Read the model definition and answer for the solid it produces. Units are mm, in the model's axes. Face numbers are marked on the shaded views. Coordinates: 2 decimals unless noted, no trailing zeros. Write each loop counter-clockwise with the first axis right and the second up, starting at its lowest first coordinate (ties: lowest second). Pieces come first, ordered by that corner, then holes. Notation, with made-up numbers: (-5, 20.5) -> (13, 20.5) arc R19 cw to (13, 51.5) -> close; hole circle Ø9 at (44, 12). An arc over 180 degrees is marked (long way). One line per item, written item: value. Start each with the question number.
from build123d import *

# Parameters (mm, degrees)
F0_R     = 9.8
F0_R_2   = 9.65
F1_DEPTH = 4
F2_DEPTH = 3
F3_R     = 0.2


with BuildPart() as f1:
    # F0 (on Top) → F1 (new body)
    with BuildSketch(Plane.XY):
        Circle(F0_R)
        Circle(F0_R_2, mode=Mode.SUBTRACT)
        Circle(F0_R_2)
    extrude(amount=F1_DEPTH)

    # F0 (on Top) → F2 (cut)
    with BuildSketch(Plane.XY):
        Circle(F0_R_2)
    extrude(amount=F2_DEPTH, mode=Mode.SUBTRACT)

    # F3
    f3_edges = [f1.edges().sort_by_distance(p)[0] for p in [
        (-9.8, 0, 4),
        (-9.65, 0, 3),
    ]]
    fillet(f3_edges, radius=F3_R)


solid = f1.part
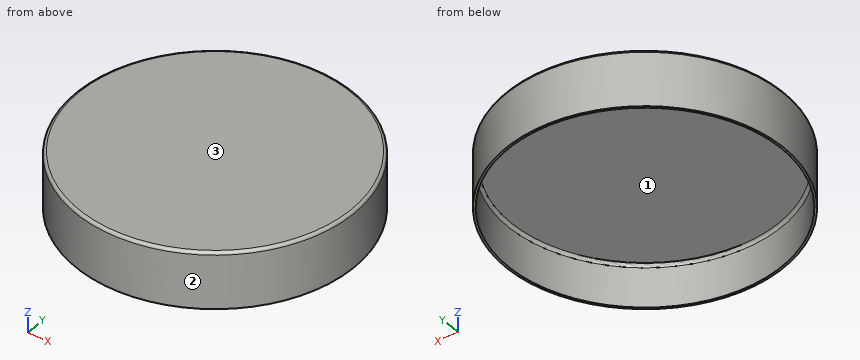
1. A cutting plane is placed at A-A on x = 0. Give the vertices of the cut face in (y, z).
2. For a pull along X with two mould halves and no side action, classify the marked faces 1, 2 and 3 as +X half, -X half, draft (parallel to the pull), parting line (faces both ways), or undercut.
3. Find the intervals of material crossed by probe 1 along Z at (x, y) = (6.5, 3.5); probe 2 along X at (y, z) = (-0.25, 2.65); probe 3 along X at (y, z) = (-8.5, 2.55), in increasing order. Write a range as from..to.
4. Given pin 1 (11.5 mm diameter, centred on x = 0, y = 0, fed in from -Z); pin 2 (1 mm diameter, centred on x = -5, z = 3, fed in from +Y); pin 3 (1 mm diameter, centred on y = -4, z = 3, fed in from -X), each flat-ended and moving along its own axis, determine where each tip first touches the part or whether it passes through.
5. A cutting plane is placed at C-C on z = 2.1. Give the vertices of the cut face in (x, y).
Derived:
1. outline: (-9.8, 0) -> (-9.65, 0) -> (-9.65, 2.8) arc R0.2 cw to (-9.45, 3) -> (9.45, 3) arc R0.2 cw to (9.65, 2.8) -> (9.65, 0) -> (9.8, 0) -> (9.8, 3.8) arc R0.2 ccw to (9.6, 4) -> (-9.6, 4) arc R0.2 ccw to (-9.8, 3.8) -> close
2. face 1: undercut
2. face 2: parting line
2. face 3: draft
3. probe 1: z = 3..4
3. probe 2: x = -9.8..-9.65, 9.65..9.8
3. probe 3: x = -4.88..-4.57, 4.57..4.88
4. pin 1: stops at z = 3
4. pin 2: stops at y = 8.71
4. pin 3: stops at x = -9.15
5. outline: circle Ø19.6 at (0, 0); hole circle Ø19.3 at (0, 0)
